Could you check a few things on this model? Use its own coordinates, in mm. Face numbers are marked on the shaded views. A direction names the side the tool comes from. Give positions to 0.01 mm unless a question says otherwise; leave off trailing zeros. Loops run counter-clockwise (first coordinate to the right, second up) from the corner with the lowest first, then second, coordinate; pieces in that order, holes last. Notation, with made-up numbers: M 24.25,-21.75 L 83.25,-21.75 A35 cw 83.25,16.25 Z; hole C 66,48 d9. An arc over 180 degrees is marked long. Return JSON: item names as keys, results as strings. Group by question number.
1. For pin 1 (3.5 mm diameter, centred on x = 42, y = 4, fed in from -Z); pin 2 (2.5 mm diameter, centred on x = 15, y = 18, fed in from +Z); pin 3 (0.6 mm diameter, centred on y = 4, z = 2.5, fed in from -X), each with a flat end and sliding along its axis, tell me the tip position at first contact or that it passes through.
2. If we section it at B-B (y = 11): Write out the boundary of the cut face in (x, z), plus the area to 3 significant figures.
3. If we section it at D-D (x = 14.5): State how many separate pieces and enclosed holes the cut face has, plus the area to 3 significant figures.
4. For the marked faces 1, 2, 3, 4 and 5, which set-ups out of +Z, -Z, +X, -X, +Y, -Y let a thin tool reach every point of the face, with its end or its side?
5. Please list where these lines run through material, in increasing order: line 1 (Y direction, x = 42, z = 3); line 2 (Y direction, x = 3, z = 1.45); line 3 (Y direction, x = 28.5, z = 2.35).
6. If we section it at A-A (x = 3): Write out the boundary of the cut face in (y, z), plus the area to 3 significant figures.
7. If we mould it in two halves opening along X, with no side actions, what happens to the marked faces 6, 7, 8 and 9? For each: +X half, -X half, draft (parallel to the pull), parting line (faces both ways), or undercut.
8. If we section it at C-C (x = 27): Write out the boundary of the cut face in (y, z).
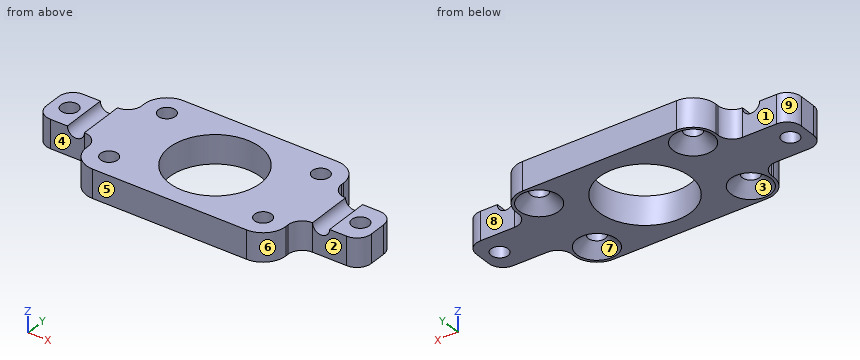
```python
from build123d import *

# Parameters (mm, degrees)
SKETCH_1_R          = 8
SKETCH_1_R_2        = 1.5
EXTRUDE_1_DEPTH     = 5
SKETCH_2_R          = 1.5
CUT_EXTRUDE_1_DEPTH = 11.5
CHAMFER_1_SIZE      = 2


with BuildPart() as part:
    # 草图1 → 凸台-拉伸1 (new body)
    with BuildSketch(Plane.XY):
        with BuildLine():
            Line((2.5, 15), (8.5, 15))
            ThreePointArc((8.5, 15), (10.267766953, 15.732233047), (11, 17.5))
            Line((11, 17.5), (11, 18))
            ThreePointArc((11, 18), (12.171572875, 20.828427125), (15, 22))
            Line((15, 22), (42, 22))
            ThreePointArc((42, 22), (44.828427125, 20.828427125), (46, 18))
            Line((46, 18), (46, 17.5))
            ThreePointArc((46, 17.5), (46.732233047, 15.732233047), (48.5, 15))
            Line((48.5, 15), (54.5, 15))
            ThreePointArc((54.5, 15), (56.267766953, 14.267766953), (57, 12.5))
            Line((57, 12.5), (57, 9.5))
            ThreePointArc((57, 9.5), (56.267766953, 7.732233047), (54.5, 7))
            Line((54.5, 7), (48.5, 7))
            ThreePointArc((48.5, 7), (46.732233047, 6.267766953), (46, 4.5))
            Line((46, 4.5), (46, 4))
            ThreePointArc((46, 4), (44.828427125, 1.171572875), (42, 0))
            Line((42, 0), (15, 0))
            ThreePointArc((15, 0), (12.171572875, 1.171572875), (11, 4))
            Line((11, 4), (11, 4.5))
            ThreePointArc((11, 4.5), (10.267766953, 6.267766953), (8.5, 7))
            Line((8.5, 7), (2.5, 7))
            ThreePointArc((2.5, 7), (0.732233047, 7.732233047), (0, 9.5))
            Line((0, 9.5), (0, 12.5))
            ThreePointArc((0, 12.5), (0.732233047, 14.267766953), (2.5, 15))
        make_face()
        with Locations((28.5, 11)):
            Circle(SKETCH_1_R, mode=Mode.SUBTRACT)
        with Locations((15, 18)):
            Circle(SKETCH_1_R_2, mode=Mode.SUBTRACT)
        with Locations(Location((15, 4, 0), (0, 0, 180))):
            Circle(SKETCH_1_R_2, mode=Mode.SUBTRACT)
        with Locations(Location((42, 18, 0), (0, 0, 180))):
            Circle(SKETCH_1_R_2, mode=Mode.SUBTRACT)
        with Locations((42, 4)):
            Circle(SKETCH_1_R_2, mode=Mode.SUBTRACT)
        with Locations((3, 11)):
            Circle(SKETCH_1_R_2, mode=Mode.SUBTRACT)
        with Locations(Location((54, 11, 0), (0, 0, 180))):
            Circle(SKETCH_1_R_2, mode=Mode.SUBTRACT)
    extrude(amount=EXTRUDE_1_DEPTH)

    # 草图2 → 切除-拉伸1 (cut)
    with BuildSketch(Plane(origin=(0, 15, 0), x_dir=(1, 0, 0), z_dir=(0, 1, 0))):
        with Locations((7, -5)):
            Circle(SKETCH_2_R)
        with Locations((50, -5)):
            Circle(SKETCH_2_R)
    extrude(amount=-CUT_EXTRUDE_1_DEPTH, mode=Mode.SUBTRACT)

    # 倒角1
    chamfer_1_edges = [part.edges().sort_by_distance(p)[0] for p in [
        (13.5, 18, 0),
        (16.5, 4, 0),
        (43.5, 18, 0),
        (40.5, 4, 0),
    ]]
    chamfer(chamfer_1_edges, length=CHAMFER_1_SIZE)


solid = part.part
```
Answer:
{
 "1": {"pin 1": "stops at z = 1.75", "pin 2": "passes through", "pin 3": "stops at x = 11"},
 "2": {"outline": "M 0,0 L 1.5,0 L 1.5,5 L 0,5 Z; M 4.5,0 L 20.5,0 L 20.5,5 L 8.5,5 A1.5 cw 5.5,5 L 4.5,5 Z; M 36.5,0 L 52.5,0 L 52.5,5 L 51.5,5 A1.5 cw 48.5,5 L 36.5,5 Z; M 55.5,0 L 57,0 L 57,5 L 55.5,5 Z", "area": "168 mm²"},
 "3": {"separate pieces": "3", "enclosed holes": "0", "area": "73.1 mm²"},
 "4": {"face 1": "+Z, -Z, -X, +Y", "face 2": "+Z, -Z, +X, -Y", "face 3": "-Z", "face 4": "+Z, -Z, -X, -Y", "face 5": "+Z, -Z, +X, -X, -Y"},
 "5": {"line 1": "y = 0 to 2.5, 5.5 to 16.5, 19.5 to 22", "line 2": "y = 7 to 9.5, 12.5 to 15", "line 3": "y = 0 to 3, 19 to 22"},
 "6": {"outline": "M 7,0 L 9.5,0 L 9.5,5 L 7,5 Z; M 12.5,0 L 15,0 L 15,5 L 12.5,5 Z", "area": "25.0 mm²"},
 "7": {"face 6": "+X half", "face 7": "undercut", "face 8": "draft", "face 9": "-X half"},
 "8": {"outline": "M 0,0 L 3.14,0 L 3.14,5 L 0,5 Z; M 18.86,0 L 22,0 L 22,5 L 18.86,5 Z"}
}
